The listing builds one solid part. Answer for the finished solid, in the listing's coordinates (mm). A direction names the side the tool comes from. Round coordinates to 2 decimals unless told otherwise and drop trailing zeros. Write each loop counter-clockwise with the first axis right and the second up, starting at its lowest first coordinate (ties: lowest second). Pieces come first, ordered by that corner, then holes. Notation, with made-up numbers: M 32.5,84 L 89.5,84 A32 ccw 89.5,120 Z; hole C 4,-34.75 d8. An arc over 180 degrees is marked long. Write each question's results on one line, items separated by ' | '.
from build123d import *

# Parameters (mm, degrees)
SKETCH4_R          = 7.9375
CUT_EXTRUDE2_DEPTH = 101.6
CHAMFER2_SIZE      = 3


with BuildPart() as part:
    # Sketch3 → Revolve1 (revolve)
    with BuildSketch(Plane.XY):
        Polygon((-11.1125, -151), (-11.1125, -41), (-12.1125, -41), (-12.1125, -16), (-5.25, -5), (-5.25, 0), (0, 0), (0, -151), align=None)
    revolve(axis=Axis((0, -151, 0), (0, 1, 0)))

    # Sketch4 → Cut-Extrude2 (cut)
    with BuildSketch(Plane.XZ.offset(151)):
        Circle(SKETCH4_R)
    extrude(amount=-CUT_EXTRUDE2_DEPTH, mode=Mode.SUBTRACT)

    # Chamfer2
    chamfer2_edges = [part.edges().sort_by_distance(p)[0] for p in [
        (11.1125, -151, 0),
    ]]
    chamfer(chamfer2_edges, length=CHAMFER2_SIZE)


solid = part.part
1) Find the intervals of material crossed by line 1 (Z direction, x = 0, y = -117.5); line 2 (Z direction, x = -6.5, y = -102); line 3 (X direction, y = -85, z = 1.75), in increasing order.
Return value:
line 1: -11.11 to -7.94, 7.94 to 11.11 | line 2: -9.01 to -4.56, 4.56 to 9.01 | line 3: -10.97 to -7.74, 7.74 to 10.97
2) The mould has two halves that part along X. Classify faces 3 (the face through (-1.72, -100.91, -7.75)), 4 (the face through (0, 0, 0)), 5 (the face through (-5, -2.5, 1.6)): +X half, -X half, draft (parallel to the pull), parting line (faces both ways), or undercut.
Return value:
face 3: undercut | face 4: draft | face 5: parting line
3) Section A-A (z = 0) is taken. Determine the outline of the cut face in (x, y), then the cut area to 3 significant figures.
Return value:
outline: M -12.11,-41 L -11.11,-41 L -11.11,-148 L -8.11,-151 L -7.94,-151 L -7.94,-49.4 L 7.94,-49.4 L 7.94,-151 L 8.11,-151 L 11.11,-148 L 11.11,-41 L 12.11,-41 L 12.11,-16 L 5.25,-5 L 5.25,0 L -5.25,0 L -5.25,-5 L -12.11,-16 Z | area: 1,670 mm²
4) Section B-B (x = 0) is taken. Determine the outline of the cut face in (y, z), then the cut area to 3 significant figures.
Return value:
outline: M -151,-8.11 L -148,-11.11 L -41,-11.11 L -41,-12.11 L -16,-12.11 L -5,-5.25 L 0,-5.25 L 0,5.25 L -5,5.25 L -16,12.11 L -41,12.11 L -41,11.11 L -148,11.11 L -151,8.11 L -151,7.94 L -49.4,7.94 L -49.4,-7.94 L -151,-7.94 Z | area: 1,670 mm²
5) Section C-C (y = -132) is taken. Determine the outline of the cut face in (x, z) (1 decimal), then the cut area to 3 significant figures.
Return value:
outline: C 0,0 d22.2; hole C 0,0 d15.9 | area: 190 mm²
6) A tool of negligible diameter and unlimited length cuts with its end or side. For faces 1 (the face through (0, -49.4, 0)), 2 (the face through (-11.553, -28.325, 3.638)), from which of +Z, -Z, +X, -X, +Y, -Y can it reach the whole face along a straight path? Write none if from no direction.
Return value:
face 1: -Y | face 2: +Y, -Y
7) Section D-D (y = -47.5) is taken. Determine the outline of the cut face in (x, z) (1 decimal), then the cut area to 3 significant figures.
Return value:
outline: C 0,0 d22.2 | area: 388 mm²
8) Each of these flat-tipped pins is pushed along its axis until it touches: pin 1 (12 mm diameter, centred on x = 0, z = -7.5, fed in from +Y); pin 2 (6 mm diameter, centred on y = -124.5, z = -1.5, fed in from +X); pin 3 (8 mm diameter, centred on x = 4.5, y = -77, fed in from -Z); pin 4 (1 mm diameter, centred on y = -82.5, z = -5, fed in from +X). Where does it stop, or does it pass through?
Return value:
pin 1: y = 0 | pin 2: x = 11.11 | pin 3: z = -11.1 | pin 4: x = 10.16
